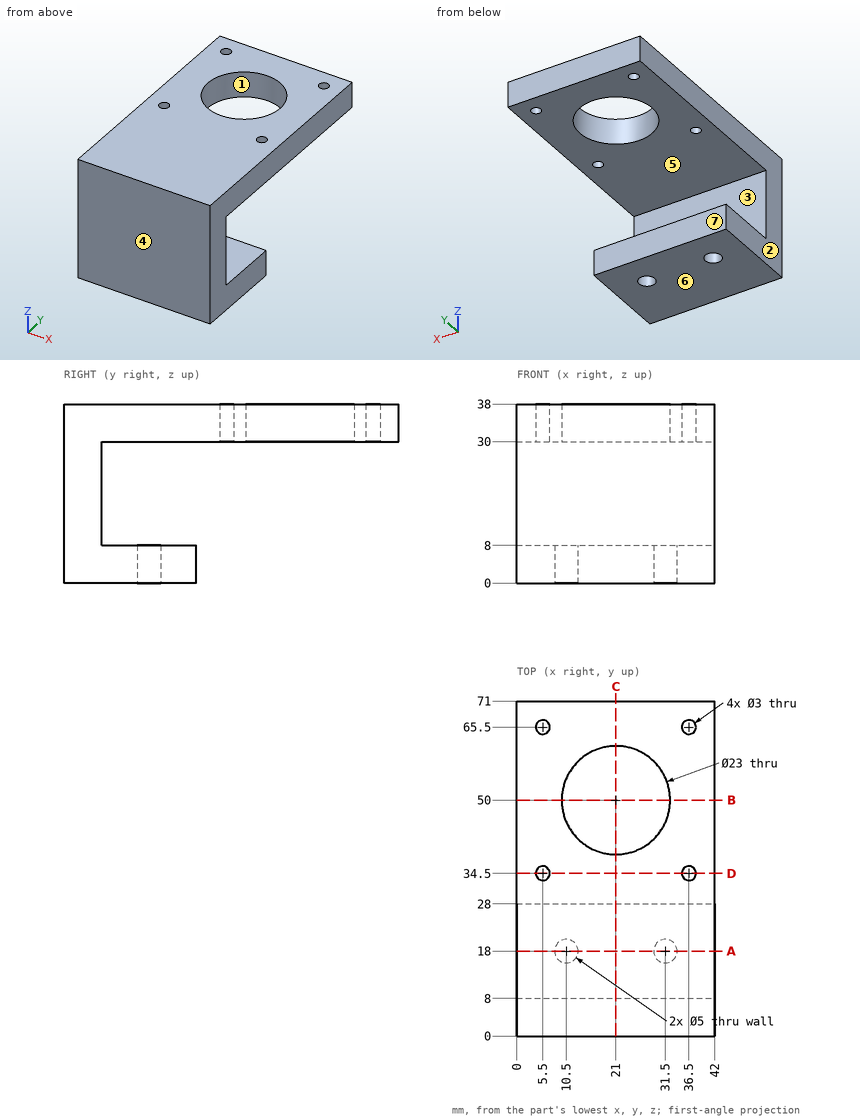
Answer from the drawing. Dimensions are ordinates in mm from the lowest x, y and z of the part. A direction names the side the tool comes from. Round coordinates to 2 decimals unless told otherwise and drop trailing zeros. Loops run counter-clockwise (first coordinate to the right, second up) from the corner with the lowest first, then second, coordinate; pieces in that order, holes last. Notation, with made-up numbers: (56, 37) - (103, 37) arc R21 ccw to (103, 43) - close; hole circle Ø9 at (-22, 27.25). An arc over 180 degrees is marked (long way). Return JSON: item names as keys, results as strings. Group by question number.
1. Which of the six approach directions +Z, -Z, +X, -X, +Y, -Y give full straight-line access (tool end or side, diameter ignored) to the marked faces 5, 6 and 7?
2. The part is cut by section B-B on y = 50. Determine the outline of the cut face in (x, z).
3. The part is cut by section C-C on x = 21. Determine the outline of the cut face in (y, z), then the cut area to 3 significant figures.
4. Each of these flat-tipped pins is pushed along its axis until it touches: P1, Ø4, axis at x = 21.5, z = 2, coming from the +Y side; P2, Ø3.5, axis at x = 5.5, y = 34.5, coming from the -Z side; P3, Ø6, axis at x = 7.5, z = 20.5, coming from the +Y side. Where does it stop, or does it pass through?
5. The part is cut by section A-A on y = 18. Determine the outline of the cut face in (x, z), then the cut area to 3 significant figures.
6. The part is cut by section D-D on y = 34.5. Determine the outline of the cut face in (x, z), then the cut area to 3 significant figures.
7. Consider probe 1 along X at (y, z) = (65.5, 33.75); probe 2 along Y at (x, z) = (5.5, 33.5); probe 3 along Z at (x, y) = (35.5, 21.5). Determine where each line is inside the solid, lowest interval first.
8. The mould has two halves that part along Y. Classify the marked faces 1, 2, 3 and 4: pulls with the +Y half, pulls with the -Y half, needs draft (parallel to the pull), parting line crosses it, or undercut.
Resolved:
{
 "1": {"face 5": "+X, -X, +Y", "face 6": "-Z, +X, -X, +Y, -Y", "face 7": "-Z, +X, -X, +Y"},
 "2": {"outline": "(0, 30) - (9.5, 30) - (9.5, 38) - (0, 38) - close; (32.5, 30) - (42, 30) - (42, 38) - (32.5, 38) - close"},
 "3": {"outline": "(0, 0) - (28, 0) - (28, 8) - (8, 8) - (8, 30) - (38.5, 30) - (38.5, 38) - (0, 38) - close; (61.5, 30) - (71, 30) - (71, 38) - (61.5, 38) - close", "area": "784 mm²"},
 "4": {"P1": "stops at y = 28", "P2": "stops at z = 30", "P3": "stops at y = 8"},
 "5": {"outline": "(0, 0) - (8, 0) - (8, 8) - (0, 8) - close; (0, 30) - (42, 30) - (42, 38) - (0, 38) - close; (13, 0) - (29, 0) - (29, 8) - (13, 8) - close; (34, 0) - (42, 0) - (42, 8) - (34, 8) - close", "area": "592 mm²"},
 "6": {"outline": "(0, 30) - (4, 30) - (4, 38) - (0, 38) - close; (7, 30) - (35, 30) - (35, 38) - (7, 38) - close; (38, 30) - (42, 30) - (42, 38) - (38, 38) - close", "area": "288 mm²"},
 "7": {"probe 1": "x = 0 to 4, 7 to 35, 38 to 42", "probe 2": "y = 0 to 33, 36 to 64, 67 to 71", "probe 3": "z = 0 to 8, 30 to 38"},
 "8": {"face 1": "undercut", "face 2": "needs draft", "face 3": "pulls with the +Y half", "face 4": "pulls with the -Y half"}
}
